```python
from build123d import *

# Parameters (mm, degrees)
F3_W            = 1.5
F3_H            = 4.2986176481
F4_DEPTH        = 8
F4_COPIES_COUNT = 3
F5_SIZE         = 1


# Not quite as in the source:
# - a pattern or mirror of a feature is missing from the dataset's text; its kind, count and spacing are read off the source's solid


with BuildPart() as f1:
    # F0 (on Front) → F1 (revolve)
    with BuildSketch(Plane.XZ):
        Polygon((-30.9, 0), (0, 0), (0, 2), (-28.9, 2), (-28.9, 12), (-30.9, 12), align=None)
    revolve(axis=Axis((0, 0, 1), (0, 0, -1)))

    # F3 (on offset) → F4 (cut)
    with BuildSketch(Plane.XY.offset(12)):
        with Locations((0, 29.3811720078)):
            Rectangle(F3_W, F3_H)
    f4 = extrude(amount=-F4_DEPTH, mode=Mode.SUBTRACT)

    # F4_copies: F4 ×3 about axis
    f4_copies_axis = Axis((0, 0, 0), (0, 0, 1))
    for i in range(1, F4_COPIES_COUNT):
        add(f4.rotate(f4_copies_axis, i * 360 / F4_COPIES_COUNT), mode=Mode.SUBTRACT)

    # F5
    f5_edges = [f1.edges().sort_by_distance(p)[0] for p in [
        (30.9, 0, 0),
    ]]
    chamfer(f5_edges, length=F5_SIZE)


solid = f1.part
```
For this review, take the finished solid that the model builds, in its own axes (mm). A direction names the side the tool comes from. Give positions to 0.01 mm unless a question says otherwise; leave off trailing zeros. Write each loop counter-clockwise with the first axis right and the second up, starting at its lowest first coordinate (ties: lowest second). Pieces come first, ordered by that corner, then holes.
Item 1: Take a section at D-D (z = 3.25). Give the boundary of the cut face in (x, y), and give its area (3 significant figures).
Item 2: Take a section at B-B (x = 0). Give the boundary of the cut face in (y, z), and give its area (3 significant figures).
Item 3: Machinability: for faces 1 (the face through (0, 0, 2)), 2 (the face through (-25.5, -15.59, 8.06)), 3 (the face through (0.75, 30, 8)), 4 (the face through (25.5, -15.59, 8.06)), which of the approach directions +Z, -Z, +X, -X, +Y, -Y give a long, thin tool a straight path to every point of the face, cutting with its end or side? Answer none if there is none.
Item 4: Take a section at C-C (y = 0). Give the boundary of the cut face in (x, z), and give its area (3 significant figures).
Item 5: Take a section at A-A (z = 10.25). Give the boundary of the cut face in (x, y), and give its area (3 significant figures).
Item 6: Insertion check: P1, Ø4, axis at x = 11.5, y = 22, coming from the +Z side; P2, Ø3, axis at y = 4.5, z = 7, coming from the +X side; P3, Ø5, axis at x = -17.5, z = 9.5, coming from the +Y side (3 decimals). Each pin has a flat end and moves straight along its axis. Give the tip position at first contact, or say it passes through.
Item 7: Wall thickness on probe 1 along X at (y, z) = (0, 6.75); probe 2 along Y at (x, z) = (0, 8.75); probe 3 along Z at (x, y) = (18.5, 3): over which ranges is each line inside the solid? List them lowest first.
Established:
1. outline: circle Ø61.8 at (0, 0); hole circle Ø57.8 at (0, 0)
1. area: 376 mm2
2. outline: (-30.9, 1) - (-29.9, 0) - (29.9, 0) - (30.9, 1) - (30.9, 4) - (28.9, 4) - (28.9, 2) - (-28.9, 2) - (-28.9, 12) - (-30.9, 12) - close
2. area: 147 mm2
3. face 1: +Z
3. face 2: +Z, -X
3. face 3: +Z, +Y
3. face 4: +Z, +X
4. outline: (-30.9, 1) - (-29.9, 0) - (29.9, 0) - (30.9, 1) - (30.9, 12) - (28.9, 12) - (28.9, 2) - (-28.9, 2) - (-28.9, 12) - (-30.9, 12) - close
4. area: 163 mm2
5. outline: (-27.13, -14.8) - (-25.39, -13.8) arc R28.9 cw to (-0.75, 28.89) - (-0.75, 30.89) arc R30.9 ccw to start; (-26.38, -16.09) arc R30.9 ccw to (26.38, -16.09) - (24.64, -15.09) arc R28.9 cw to (-24.64, -15.09) - close; (0.75, 28.89) arc R28.9 cw to (25.39, -13.8) - (27.13, -14.8) arc R30.9 ccw to (0.75, 30.89) - close
5. area: 367 mm2
6. P1: stops at z = 2
6. P2: stops at x = 30.75
6. P3: stops at y = 27.015
7. probe 1: x = -30.9 to -28.9, 28.9 to 30.9
7. probe 2: y = -30.9 to -28.9
7. probe 3: z = 0 to 2
